```python
from build123d import *

# Parameters (mm, degrees)
F0_W     = 15.5
F0_H     = 15
F1_DEPTH = 2
F3_R     = 1
F3_R_2   = 1.0194429363
F4_DEPTH = 2
F5_W     = 5
F5_H     = 7
F6_DEPTH = 2


# Not quite as in the source:
# - a feature names something its author has since deleted; it is built from what else it names


with BuildPart() as f1:
    # F0 (on Top) → F1 (new body)
    with BuildSketch(Plane.XY):
        Rectangle(F0_W, F0_H)
    extrude(amount=F1_DEPTH)

    # F3 (on offset) → F4 (cut)
    with BuildSketch(Plane.XY.offset(2)):
        with Locations((5.75, 6)):
            Circle(F3_R)
        with Locations((5.6829168866, 3.0007501178)):
            Circle(F3_R)
        with Locations((5.7305570637, -0.0183169664)):
            Circle(F3_R_2)
        with Locations((5.7305570637, 0.0183169664)):
            Circle(F3_R_2)
        with Locations((5.6829168866, -3.0007501178)):
            Circle(F3_R)
        with Locations((5.75, -6)):
            Circle(F3_R)
    extrude(amount=-F4_DEPTH, mode=Mode.SUBTRACT)

    # F5 (on offset) → F6 (join)
    with BuildSketch(Plane.XY.offset(2)):
        with Locations((-6.75, 0)):
            Rectangle(F5_W, F5_H)
    extrude(amount=F6_DEPTH)


solid = f1.part
```
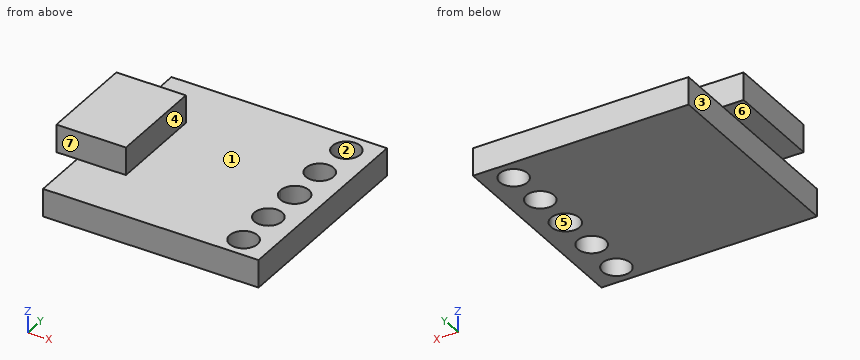
Verification items for the finished model (mm, model axes). Face numbers are marked on the shaded views. A direction names the side the tool comes from. Give positions to 0.01 mm unless a question says otherwise; leave off trailing zeros. Order: outer loops, then holes, each group sorted by start corner. A loop starts at its lowest first (then second) coordinate and runs counter-clockwise, first axis right, second up. Notation, with made-up numbers: (16, 29) -> (43, 29) arc R31 ccw to (43, 64) -> close; hole circle Ø11 at (70.25, 37). An arc over 180 degrees is marked (long way). One line per item, written item: value.
(1) Sectioned sample at A-A on y = -6. Record the cut outline in (x, z).
Final values:
outline: (-7.75, 0) -> (4.75, 0) -> (4.75, 2) -> (-7.75, 2) -> close; (6.75, 0) -> (7.75, 0) -> (7.75, 2) -> (6.75, 2) -> close
(2) Sectioned sample at B-B on x = -7.5. Record the cut outline in (y, z).
Final values:
outline: (-7.5, 0) -> (7.5, 0) -> (7.5, 2) -> (3.5, 2) -> (3.5, 4) -> (-3.5, 4) -> (-3.5, 2) -> (-7.5, 2) -> close
(3) Sectioned sample at C-C on y = -1.75. Record the cut outline in (x, z), then the cut area to 3 significant figures.
Final values:
outline: (-9.25, 2) -> (-7.75, 2) -> (-7.75, 0) -> (7.75, 0) -> (7.75, 2) -> (-4.25, 2) -> (-4.25, 4) -> (-9.25, 4) -> close
area: 41.0 mm^2
(4) Sectioned sample at D-D on x = 5.75. Record the cut outline in (y, z), then the cut area to 3 significant figures.
Final values:
outline: (-7.5, 0) -> (-7, 0) -> (-7, 2) -> (-7.5, 2) -> close; (-5, 0) -> (-4, 0) -> (-4, 2) -> (-5, 2) -> close; (-2, 0) -> (-1.04, 0) -> (-1.04, 2) -> (-2, 2) -> close; (1.04, 0) -> (2, 0) -> (2, 2) -> (1.04, 2) -> close; (4, 0) -> (5, 0) -> (5, 2) -> (4, 2) -> close; (7, 0) -> (7.5, 0) -> (7.5, 2) -> (7, 2) -> close
area: 9.87 mm^2
(5) Draft check along X on the marked faces 1, 2, 3 and 4. Enter one of: pulls with the +X half, pulls with the -X half, needs draft (parallel to the pull), parting line crosses it, or undercut.
Final values:
face 1: needs draft
face 2: undercut
face 3: pulls with the -X half
face 4: pulls with the +X half
(6) Gauge pin test, flat ends, axial feed: pin 1 (1 mm diameter, centred on x = -8, z = 2.5, fed in from +Y); pin 2 (2.5 mm diameter, centred on x = 5.68, y = 3, fed in from +Z); pin 3 (1.2 mm diameter, centred on x = -8.5, y = -0.5, fed in from -Z). Record the tip position at first contact, or that the pin passes through.
Final values:
pin 1: y = 3.5
pin 2: z = 2
pin 3: z = 2
(7) Scan lines: line 1 along X through (y, z) = (-1, 3.15); line 2 along Z through (x, y) = (-4, -1.75); line 3 along X through (y, z) = (-5.25, 1.2). Record each from-to range of solid material in increasing order. Write a range as [from, to].
Final values:
line 1: [-9.25, -4.25]
line 2: [0, 2]
line 3: [-7.75, 5.09], [6.41, 7.75]
(8) Tool access check on the marked faces 5, 6 and 7. Record the directions out of +Z, -Z, +X, -X, +Y, -Y that give a thin tool (end or side, any length) a straight path to the whole face; none if there is none.
Final values:
face 5: +Z, -Z
face 6: -Z, -X, +Y, -Y
face 7: +Z, +X, -X, -Y
